Model file for the job. Use its own axes, mm. Face numbers are marked on the shaded views. Round coordinates to 2 decimals unless told otherwise and drop trailing zeros. Order: outer loops, then holes, each group sorted by start corner. A loop starts at its lowest first (then second) coordinate and runs counter-clockwise, first axis right, second up. Notation, with made-up numbers: (30.25, -27) -> (83.25, -27) arc R30 ccw to (83.25, -4) -> close; hole circle Ø2 at (41.5, 24). An arc over 180 degrees is marked (long way). Use CSV: the item, a comma, the result in double quotes.
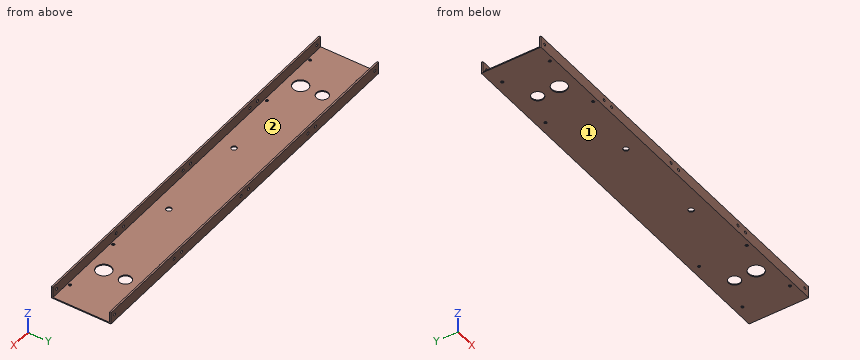
```python
from build123d import *

# Parameters (mm, degrees)
SKETCH_1_W          = 720
SKETCH_1_H          = 110
SKETCH_1_R          = 11
SKETCH_1_R_2        = 14
SKETCH_1_R_3        = 2.5
SKETCH_1_R_4        = 5
EXTRUDE_1_DEPTH     = 2
SKETCH_2_W          = 720
SKETCH_2_H          = 3
EXTRUDE_2_DEPTH     = 20
SKETCH_3_R          = 2.5
CUT_EXTRUDE_3_DEPTH = 114


with BuildPart() as part:
    # 草图1 → 凸台-拉伸1 (new body)
    with BuildSketch(Plane.XY):
        with Locations((266.780748393, 19.519407272)):
            Rectangle(SKETCH_1_W, SKETCH_1_H)
        with Locations((529.466526581, 34.519407272)):
            Circle(SKETCH_1_R, mode=Mode.SUBTRACT)
        with Locations((0, 34.519407272)):
            Circle(SKETCH_1_R, mode=Mode.SUBTRACT)
        with Locations((0, -5.480592728)):
            Circle(SKETCH_1_R_2, mode=Mode.SUBTRACT)
        with Locations((58.117699254, -27.930592728)):
            Circle(SKETCH_1_R_3, mode=Mode.SUBTRACT)
        with Locations((58.25, 59.969407272)):
            Circle(SKETCH_1_R_3, mode=Mode.SUBTRACT)
        with Locations((-58.25, 59.969407272)):
            Circle(SKETCH_1_R_3, mode=Mode.SUBTRACT)
        with Locations((179.094970205, -5.480592728)):
            Circle(SKETCH_1_R_4, mode=Mode.SUBTRACT)
        with Locations((354.466526581, -5.480592728)):
            Circle(SKETCH_1_R_4, mode=Mode.SUBTRACT)
        with Locations((-58.25, -27.930592728)):
            Circle(SKETCH_1_R_3, mode=Mode.SUBTRACT)
        with Locations((529.466526581, -5.480592728)):
            Circle(SKETCH_1_R_2, mode=Mode.SUBTRACT)
        with Locations((587.584225835, -27.930592728)):
            Circle(SKETCH_1_R_3, mode=Mode.SUBTRACT)
        with Locations((587.716526581, 59.969407272)):
            Circle(SKETCH_1_R_3, mode=Mode.SUBTRACT)
        with Locations((471.216526581, 59.969407272)):
            Circle(SKETCH_1_R_3, mode=Mode.SUBTRACT)
        with Locations((471.216526582, -27.930592728)):
            Circle(SKETCH_1_R_3, mode=Mode.SUBTRACT)
    extrude(amount=EXTRUDE_1_DEPTH)

    # 草图2 → 凸台-拉伸2 (add)
    with BuildSketch(Plane.XY.offset(2)):
        with Locations((266.780748393, 73.019407272)):
            Rectangle(SKETCH_2_W, SKETCH_2_H)
        with Locations((266.780748393, -33.980592728)):
            Rectangle(SKETCH_2_W, SKETCH_2_H)
    extrude(amount=EXTRUDE_2_DEPTH)

    # 草图3 → 切除-拉伸3 (cut)
    with BuildSketch(Plane(origin=(0, 74.519407272, 0), x_dir=(1, 0, 0), z_dir=(0, 1, 0))):
        with Locations(Location((456.780748393, -12, 0), (0, 0, 270))):
            Circle(SKETCH_3_R)
        with Locations(Location((616.780748393, -12, 0), (0, 0, 270))):
            Circle(SKETCH_3_R)
        with Locations(Location((436.780748393, -12, 0), (0, 0, 270))):
            Circle(SKETCH_3_R)
        with Locations(Location((276.780748393, -12, 0), (0, 0, 270))):
            Circle(SKETCH_3_R)
        with Locations(Location((256.780748393, -12, 0), (0, 0, 270))):
            Circle(SKETCH_3_R)
        with Locations(Location((96.780748393, -12, 0), (0, 0, 270))):
            Circle(SKETCH_3_R)
        with Locations(Location((76.780748393, -12, 0), (0, 0, 270))):
            Circle(SKETCH_3_R)
        with Locations(Location((-83.219251607, -12, 0), (0, 0, 270))):
            Circle(SKETCH_3_R)
    extrude(amount=-CUT_EXTRUDE_3_DEPTH, mode=Mode.SUBTRACT)


solid = part.part
```
Q1. Mould opens along Y. For the marked faces 1 and 2 say: +Y half, -Y half, draft (parallel to the pull), parting line (faces both ways), or undercut.
From the geometry:
face 1,"draft"
face 2,"undercut"
Q2. Cut at A-A (x = 0). Give the cut face in (y, z), plus the area to 3 significant figures.
From the geometry:
outline,"(-35.48, 0) -> (-19.48, 0) -> (-19.48, 2) -> (-32.48, 2) -> (-32.48, 22) -> (-35.48, 22) -> close; (8.52, 0) -> (23.52, 0) -> (23.52, 2) -> (8.52, 2) -> close; (45.52, 0) -> (74.52, 0) -> (74.52, 22) -> (71.52, 22) -> (71.52, 2) -> (45.52, 2) -> close"
area,"240 mm²"
Q3. Pin check, flat tips, straight feed: pin 1 (6.5 mm diameter, centred on x = 96.78, z = 12, fed in from -Y); pin 2 (4 mm diameter, centred on x = 21.5, y = -22, fed in from +Z). Stop position of each tip, or through.
From the geometry:
pin 1,"stops at y = -35.48"
pin 2,"stops at z = 2"
Q4. Probe line 1 along Y through (x, z) = (58.25, 1.4); line 2 along Y through (x, z) = (157, 12.25); line 3 along Z through (x, y) = (201, 48.5). List the from-to ranges inside material, lowest first.
From the geometry:
line 1,"y = -35.48 to -30.43, -25.43 to 57.47, 62.47 to 74.52"
line 2,"y = -35.48 to -32.48, 71.52 to 74.52"
line 3,"z = 0 to 2"
